Build history of the part. All positions in model axes, mm. Face numbers are marked on the shaded views. A direction names the side the tool comes from. Give positions to 0.01 mm unless a question says otherwise; leave off trailing zeros. Order: outer loops, then holes, each group sorted by start corner. A loop starts at its lowest first (then second) coordinate and runs counter-clockwise, first axis right, second up. Notation, with made-up numbers: (39.25, 88) - (78.25, 88) arc R27 cw to (78.25, 109) - close; hole circle Ø5 at (62, 26.5). An arc over 180 degrees is marked (long way). Use a Markdown table: item, result. Add a question column.
(1) Wall check: line 1 (X direction, y = 15.45, z = -65.8); line 2 (Z direction, x = 0, y = 15.25); line 3 (X direction, y = 10.75, z = -24.5). Give the ranges that are in metal, low to high.
(2) Slice it at C-C (x = 19). Write the cut outline in (y, z), then the cut area to 3 significant figures.
(3) Which spindle directions (+Z, -Z, +X, -X, +Y, -Y) get a long thin tool onto all of the face, cutting with end or side? Do the marked faces 1 and 2. Say none if no direction does.
(4) Slice it at A-A (z = -65.8). Write the cut outline in (x, y), then the cut area to 3 significant figures.
(5) Slice it at B-B (x = 0). Write the cut outline in (y, z).
(6) Flat gauge pins, fed straight in: pin 1 (0.5 mm diameter, centred on x = 46, y = 6, fed in from +Z); pin 2 (1.5 mm diameter, centred on y = 16.5, z = -63, fed in from -X); pin 3 (1.5 mm diameter, centred on y = 16.5, z = -63, fed in from +X). Where does each tip first touch, or does it go through?
(7) Mould opens along X. For the marked faces 3, 4 and 5 say: +X half, -X half, draft (parallel to the pull), parting line (faces both ways), or undercut.
(8) Slice it at D-D (z = 38). Write the cut outline in (x, y).
Autodesk Inventor part; units mm, degrees
ref_plane "YZ Plane" through (0, 0, 0) normal (1, 0, 0) x (0, 1, 0)
ref_plane "XZ Plane" through (0, 0, 0) normal (0, 1, 0) x (-1, 0, 0)
ref_plane "XY Plane" through (0, 0, 0) normal (0, 0, 1) x (1, 0, 0)
sketch "Sketch1" plane through (0, 0, 0) normal (0, 1, 0) x (-1, 0, 0)
  line L0 (50, -60) -> (-50, -60)
  line L1 (-50, -60) -> (-50, 60)
  line L2 (-50, 60) -> (50, 60)
  line L3 (50, 60) -> (50, -60)
  line L4 (50, -60) -> (-50, 60) construction
  line L5 (-50, -60) -> (50, 60) construction
  point P0 (0, 0)
  dimension "d0" = 100
  dimension "d1" = 120
extrude "Extrusion1" add sketch "Sketch1" along normal blind 26
sketch "Sketch2" plane through (0, 26, 0) normal (0, 1, 0) x (1, 0, 0)
  line L0 (-41, -60) -> (41, -60)
  line L1 (-50, -60) -> (50, -60)
  line L2 (41, -60) -> (41, -4.7988)
  line L3 (50, 60) -> (-50, 60)
  line L4 (-41, -60) -> (-41, 55)
  line L5 (-41, 55) -> (41, 55)
  line L6 (41, 55) -> (41, -4.7988)
  point P0 (0, 0)
  dimension "d23" = 115
extrude "Extrusion2" cut sketch "Sketch2" against normal through all
sketch "Sketch11" plane through (0, 0, 0) normal (0, -1, 0) x (1, 0, 0)
  arc A0 (46, -10.5) -> (-46, -10.5) centre (0, -10.5) ccw
  line L0 (41, -55) -> (-41, -55)
  line L1 (-46, -10.5) -> (46, -10.5)
  line L2 (46, -10.5) -> (46, -55)
  line L3 (46, -55) -> (-46, -55)
  line L4 (-46, -55) -> (-46, -10.5)
  point P0 (0, 0)
  dimension "d24" = 92
  dimension "d25" = 44.5
extrude "Extrusion7" cut sketch "Sketch11" against normal blind 5.4
sketch "Sketch13" plane through (-41, 26, 60) normal (1, 0, 0) x (0, 0, -1)
  line L0 (0, -26) -> (0, 0)
  line L1 (0, -24) -> (115.5309, -24)
  line L2 (115.5309, -24) -> (115.5309, -20.6)
  line L3 (115.5309, -20.6) -> (0, -20.6)
  line L4 (0, -20.6) -> (0, -24)
  line L5 (49.6433, -26) -> (0, -26)
  point P0 (60, -26)
  point P1 (0, -20.6)
  dimension "d48" = 115.5309
  dimension "d49" = 3.4
  dimension "d50" = 2
extrude "Extrusion8" cut sketch "Sketch13" against normal through all both and the other way through all
sketch "Sketch14" plane through (-41, 26, 60) normal (1, 0, 0) x (0, 0, -1)
  line L0 (0, -20.6) -> (0, 0)
  line L1 (0, 0) -> (49.643, 0)
  line L2 (49.643, 0) -> (49.643, -20.6)
  line L3 (49.643, -20.6) -> (0, -20.6)
  line L4 (0, -20.6) -> (0, 0)
  point P0 (60, -26)
  dimension "d51" = 20.6
  dimension "d52" = 49.643
extrude "Extrusion9" cut sketch "Sketch14" along normal through all both and the other way through all
sketch "Sketch15" plane through (0, 0, 0) normal (1, 0, 0) x (0, 1, 0)
  line L0 (26, -55) -> (5.4, -55)
  line L1 (7, 10.357) -> (26, -55)
  line L2 (26, -55) -> (26, 10.357)
  line L3 (26, 10.357) -> (7, 10.357)
  point P0 (0, 0)
  dimension "d53" = 65.357
  dimension "d54" = 19
extrude "Extrusion10" cut sketch "Sketch15" against normal through all both and the other way through all
fillet "Fillet1" radius 5 4 edges at (-41, 15.7, -55) (50, 13, -60) (-50, 13, -60) (41, 15.7, -55)
fillet "Fillet2" radius 5 2 edges at (-46, 1, -55) (46, 1, -55)
sketch "Sketch16" plane through (45, 0, -60) normal (0, 0, -1) x (-1, 0, 0)
  line L0 (45, 0) -> (45, 26)
  line L1 (81, 26) -> (9, 26)
  line L2 (40.8, 17.5345) -> (49.2, 17.5345)
  line L3 (49.2, 17.5345) -> (49.2, 14.5345)
  line L4 (49.2, 14.5345) -> (40.8, 14.5345)
  line L5 (40.8, 14.5345) -> (40.8, 17.5345)
  line L6 (40.8, 17.5345) -> (49.2, 14.5345) construction
  line L7 (49.2, 17.5345) -> (40.8, 14.5345) construction
  point P0 (45, 16.0345)
  dimension "d38" = 8.4
  dimension "d39" = 3
extrude "Extrusion11" add sketch "Sketch16" along normal blind 10
sketch "Sketch17" plane through (-4.2, 17.5345, -60) normal (0, 1, 0) x (1, 0, 0)
  circle A0 centre (4.2, 5.8) radius 2.7
  line L0 (0, 0) -> (0, 10)
  line L1 (0, 10) -> (8.4, 10)
  point P0 (4.2, -60)
  dimension "d42" = 5.4
  dimension "d43" = 4.2
  dimension "d44" = 4.2
extrude "Extrusion12" cut sketch "Sketch17" against normal through all
fillet "Fillet5" radius 2 2 edges at (-4.2, 16.0345, -70) (4.2, 16.0345, -70)
sketch "Sketch18" plane through (45, 0, -60) normal (0, 0, -1) x (-1, 0, 0)
  point P0 (45, 0)
sketch "Sketch19" plane through (-50, 5.4, -55) normal (-1, 0, 0) x (0, 0, 1)
  point P0 (55, -5.4)
sketch "Sketch20" plane through (-50, 0, 60) normal (0, 0, 1) x (1, 0, 0)
  line L0 (9, 2) -> (0, 2)
  line L1 (0, 0) -> (9, 0)
  line L2 (0, 2) -> (9, 2)
  line L3 (9, 2) -> (9, 0)
  line L4 (9, 0) -> (0, 0)
  line L5 (0, 0) -> (0, 2)
  line L6 (100, 0) -> (95, 0)
  line L7 (100, 2) -> (91, 2)
  line L8 (100, 0) -> (91, 0)
  line L9 (91, 0) -> (91, 2)
  line L10 (91, 2) -> (100, 2)
  line L11 (100, 2) -> (100, 0)
  point P0 (50, 0)
extrude "Extrusion13" add sketch "Sketch20" along normal blind 15
fillet "Fillet7" radius 2 4 edges at (-41, 6.2, 10.357) (-50, 6.2, 10.357) (50, 6.2, 10.357) (41, 6.2, 10.357)
fillet "Fillet8" radius 2 4 edges at (50, 1, 75) (41, 1, 75) (-41, 1, 75) (-50, 1, 75)
properties part number "Khay gạt cốc"
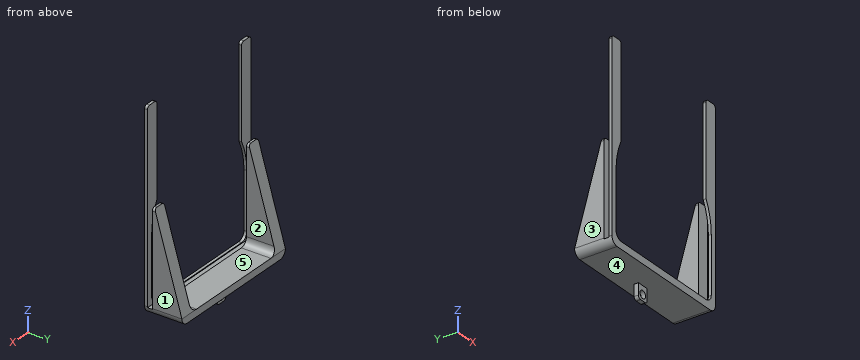
Solution:
| question | item | result |
|---|---|---|
| 1 | line 1 | -4.2 to -2.7, 2.7 to 4.2 |
| 1 | line 2 | -70 to -68.5, -63.1 to -55 |
| 1 | line 3 | -50 to -41, 41 to 50 |
| 2 | outline | (0, -60) - (26, -60) - (26, -55) - (5.4, -55) - (5.4, -55.53) - (2, -55.53) - (2, -55) - (0, -55) - close |
| 2 | area | 128 mm2 |
| 3 | face 1 | +Z, -Z, +X, +Y, -Y |
| 3 | face 2 | +Z, +Y, -Y |
| 4 | outline | (-4.2, 14.53) - (-2.7, 14.53) - (-2.7, 17.53) - (-4.2, 17.53) - close; (2.7, 14.53) - (4.2, 14.53) - (4.2, 17.53) - (2.7, 17.53) - close |
| 4 | area | 9.00 mm2 |
| 5 | outline | (0, -60) - (14.53, -60) - (14.53, -63.1) - (17.53, -63.1) - (17.53, -60) - (26, -60) - (26, -55) - (5.4, -55) - (5.4, -55.53) - (2, -55.53) - (2, -55) - (0, -55) - close; (14.53, -70) - (17.53, -70) - (17.53, -68.5) - (14.53, -68.5) - close |
| 6 | pin 1 | z = 10.36 |
| 6 | pin 2 | x = -4.2 |
| 6 | pin 3 | x = 4.2 |
| 7 | face 3 | -X half |
| 7 | face 4 | draft |
| 7 | face 5 | undercut |
| 8 | outline | (-50, 0) - (-41, 0) - (-41, 2) - (-50, 2) - close; (41, 0) - (50, 0) - (50, 2) - (41, 2) - close |
